```python
from build123d import *

# Parameters (mm, degrees)
SKIZZE1_W                                 = 25
SKIZZE1_H                                 = 24
PCB_DEPTH                                 = 0.9
SKIZZE2_R                                 = 1.05
MOUNTING_HOLES_DEPTH                      = 20.165333287
SKIZZE3_W                                 = 20.8
SKIZZE3_H                                 = 5.5
CONNECTOR_CLOSED_DEPTH                    = 2.4
SKIZZE4_W                                 = 17.7
SKIZZE4_H                                 = 11.6
COMPONENTS_WORST_CASE_BOUNDARY_BOX_DEPTH  = 1.3
CABLE_156MM_FREE_LENGTH_START             = -8
CABLE_156MM_FREE_LENGTH_DEPTH             = 16
SKIZZE7_W                                 = 3
SKIZZE7_H                                 = 2
COMPONENTS_WORST_CASE_BOUNDARY_BOX2_DEPTH = 0.6
SKIZZE8_W                                 = 1.3
SKIZZE8_H                                 = 0.9
STATUS_LED_DEPTH                          = 0.01


# Read off the part's stored shape, not the designer's step: Cable_156mm_free_Length
with BuildPart() as part:
    # Skizze1 → PCB (new body)
    with BuildSketch(Plane(origin=(0, 0, 0), x_dir=(1, 0, 0), z_dir=(0, 1, 0))):
        with Locations((0, 2.5)):
            Rectangle(SKIZZE1_W, SKIZZE1_H)
    extrude(amount=-PCB_DEPTH)

    # Skizze2 → Mounting_Holes (cut, through all)
    with BuildSketch(Plane(origin=(0, 0, 0), x_dir=(1, 0, 0), z_dir=(0, 1, 0))):
        with Locations(Location((10.5, 12.5, 0), (0, 0, 270))):
            Circle(SKIZZE2_R)
        with Locations(Location((10.5, 0, 0), (0, 0, 270))):
            Circle(SKIZZE2_R)
        with Locations(Location((-10.5, 0, 0), (0, 0, 90))):
            Circle(SKIZZE2_R)
        with Locations(Location((-10.5, 12.5, 0), (0, 0, 90))):
            Circle(SKIZZE2_R)
    extrude(amount=-MOUNTING_HOLES_DEPTH, mode=Mode.SUBTRACT)

    # Skizze3 → Connector_closed (add)
    with BuildSketch(Plane.XZ.offset(0.9)):
        with Locations((0, 6.75)):
            Rectangle(SKIZZE3_W, SKIZZE3_H)
    extrude(amount=CONNECTOR_CLOSED_DEPTH)

    # Skizze4 → Components_worst-case_Boundary-Box (add)
    with BuildSketch(Plane.XZ.offset(0.9)):
        with Locations((-0.15, -6.7)):
            Rectangle(SKIZZE4_W, SKIZZE4_H)
    extrude(amount=COMPONENTS_WORST_CASE_BOUNDARY_BOX_DEPTH)

    # Cable_156mm_free_Length outline → Cable_156mm_free_Length (add)
    with BuildSketch(Plane.YZ.offset(CABLE_156MM_FREE_LENGTH_START)):
        with BuildLine():
            add(Edge.make_bspline(
                [(-2.5, 9.5), (-2.475225113, 12.836586164), (-2.435306032, 18.21273383), (-1.780893788, 25.199891819), (-0.848086938, 32.316273634), (-1.279790623, 43.443994082), (-0.388416893, 60.791916601), (1.903305425, 83.198557796), (3.468421225, 108.473808964), (3.57358047, 134.366469325), (-0.398617572, 150.91775474), (-2.311961718, 158.890243708)],
                knots=[0, 0, 0, 0, 0.066565355, 0.107254889, 0.139591388, 0.210160277, 0.329584285, 0.485565806, 0.660213078, 0.836330084, 1, 1, 1, 1], degree=3))
            Line((-2.5, 9.5), (-2.1, 9.5))
            add(Edge.make_bspline(
                [(-2.1, 9.5), (-2.074945976, 12.831496447), (-2.03457713, 18.199443194), (-1.385285743, 25.13899131), (-0.448711873, 32.285274364), (-0.878853095, 43.46148369), (0.008252641, 60.724222754), (2.300661353, 83.153569069), (3.867117874, 108.441464768), (3.977764902, 134.372552415), (-0.006644422, 150.991885803), (-1.925870548, 158.99715239)],
                knots=[0, 0, 0, 0, 0.066565355, 0.107254889, 0.139591388, 0.210160277, 0.329584285, 0.485565806, 0.660213078, 0.836330084, 1, 1, 1, 1], degree=3))
            Line((-1.925870548, 158.99715239), (-3.203138794, 164.859625062))
            Line((-3.203138794, 164.859625062), (-3.593970306, 164.774473846))
            Line((-3.593970306, 164.774473846), (-2.311961718, 158.890243708))
        make_face()
    extrude(amount=CABLE_156MM_FREE_LENGTH_DEPTH)

    # Skizze7 → Components_worst-case_Boundary-Box2 (add)
    with BuildSketch(Plane(origin=(0, 0, 0), x_dir=(1, 0, 0), z_dir=(0, 1, 0))):
        with Locations((7, 9.9)):
            Rectangle(SKIZZE7_W, SKIZZE7_H)
    extrude(amount=COMPONENTS_WORST_CASE_BOUNDARY_BOX2_DEPTH)

    # Skizze8 → Status_LED (cut)
    with BuildSketch(Plane(origin=(0, 0.6, 0), x_dir=(1, 0, 0), z_dir=(0, 1, 0))):
        with Locations((7.45, 9.45)):
            Rectangle(SKIZZE8_W, SKIZZE8_H)
    extrude(amount=-STATUS_LED_DEPTH, mode=Mode.SUBTRACT)


solid = part.part
```
Here's how the part is built. I have some questions about the finished solid (model axes, mm). A direction names the side the tool comes from. Coordinates: 2 decimals unless noted, no trailing zeros. One line per item, written item: value.
1. On a 3-axis mill with a long thin cutter (end or side, diameter ignored), from which of +Z, -Z, +X, -X, +Y, -Y can I reach the whole of each face in a straight line? I mean faces 1 (the flat face through (-8, 2.7, 93.3)), 2 (the flat face through (8, 2.7, 93.3)), 3 (the flat face through (0, -2.2, -7)). Say none if no direction works.
Geometry says:
face 1: +Z, -X, +Y, -Y
face 2: +Z, +X, +Y, -Y
face 3: -Z, +X, -X, -Y
2. Thinking about a two-plate mould opening in Z: for faces 4 (the flat face through (0, -0.9, 0)), 5 (the flat face through (0, -3.3, 7)), 6 (the flat face through (-0.112, -2.556, 161.887)), which applies, +Z half, -Z half, draft (parallel to the pull), parting line (faces both ways), or undercut?
Geometry says:
face 4: undercut
face 5: draft
face 6: +Z half
3. Will these pins go through, and if not, where does the flat tip stop? pin 1 Ø3 at (x, y) = (-0.5, 1) entering from -Z; pin 2 Ø1.6 at (x, z) = (-2, 5.5) entering from -Y; pin 3 Ø1.7 at (x, z) = (-10.5, -12.5) entering from -Y; pin 4 Ø3 at (x, z) = (-6.5, 3.5) entering from +Y.
Geometry says:
pin 1: stops at z = -14.5
pin 2: stops at y = -3.3
pin 3: passes through
pin 4: stops at y = 0
4. Please list where these lines run through material, in increasing order: probe 1 along X at (y, z) = (-0.6, 0); probe 2 along Z at (x, y) = (-10.5, -0.5); probe 3 along Z at (x, y) = (8.25, -1.25).
Geometry says:
probe 1: x = -12.5 to -11.55, -9.45 to 9.45, 11.55 to 12.5
probe 2: z = -14.5 to -13.55, -11.45 to -1.05, 1.05 to 9.5
probe 3: z = -12.5 to -0.9, 4 to 9.5
